from build123d import *

# Parameters (mm, degrees)
SKETCH1_R           = 7.9375
BOSS_EXTRUDE1_DEPTH = 19.05
SKETCH2_W           = 3.175
SKETCH2_H           = 3.446915699
BOSS_EXTRUDE2_DEPTH = 19.05
SKETCH3_R           = 5.5626
CUT_EXTRUDE1_DEPTH  = 19.05


with BuildPart() as part:
    # Sketch1 → Boss-Extrude1 (new body)
    with BuildSketch(Plane(origin=(0, 0, 0), x_dir=(0, 0, -1), z_dir=(1, 0, 0))):
        Circle(SKETCH1_R)
    extrude(amount=BOSS_EXTRUDE1_DEPTH)

    # Sketch2 → Boss-Extrude2 (add)
    with BuildSketch(Plane.ZY):
        with Locations((0, 7.636442151)):
            Rectangle(SKETCH2_W, SKETCH2_H)
        with Locations((0, -7.636442151)):
            Rectangle(SKETCH2_W, SKETCH2_H)
    extrude(amount=-BOSS_EXTRUDE2_DEPTH)

    # Sketch3 → Cut-Extrude1 (cut)
    with BuildSketch(Plane.ZY):
        Circle(SKETCH3_R)
    extrude(amount=-CUT_EXTRUDE1_DEPTH, mode=Mode.SUBTRACT)


solid = part.part
For this review, take the finished solid that the model builds, in its own axes (mm). A direction names the side the tool comes from. Round coordinates to 2 decimals unless told otherwise and drop trailing zeros. Order: outer loops, then holes, each group sorted by start corner. A loop starts at its lowest first (then second) coordinate and runs counter-clockwise, first axis right, second up. Notation, with made-up numbers: M 19.25,52 L 61.25,52 A13 ccw 61.25,63 Z; hole C 14.5,-15.75 d8. An arc over 180 degrees is marked long. Write each question's results on one line, items separated by ' | '. Start each with the question number.
1. Add section B-B (y = 0). State the section outline as (x, z) points, then the cut area to 3 significant figures.
2. Add section A-A (z = 0). State the section outline as (x, y) points.
3. To check wall thickness, follow L1, parallel to Y at x = 13, z = 0; L2, parallel to Z at x = 6.5, y = -0.25; L3, parallel to Z at x = 6.75, y = -8.5. State the ranges of each line that lie inside material, in increasing order. Write a range as [from, to].
4. Add section D-D (y = -6.75). State the section outline as (x, z) points, then the cut area to 3 significant figures.
5. Draft analysis for pull direction Z (two halves, no side actions). For faces 4 (the face through (9, 9, -1.588)), 5 (the face through (9, -9, 1.588)), 6 (the face through (9.392, 1.671, 5.306)), state which applies: pulls with the +Z half, pulls with the -Z half, needs draft (parallel to the pull), parting line crosses it, or undercut.
6. Tool access review of faces 1 (the face through (9, -9, -1.588)), 2 (the face through (9, 9, 1.588)), 3 (the face through (9.392, 0.152, 7.936)): name each direction out of +Z, -Z, +X, -X, +Y, -Y from which nothing blocks a thin tool from reaching the whole face with its end or side.
7. Clearance check with flat-ended pins moving along their axes: pin 1 Ø1 at (x, z) = (16.5, 6) entering from +Y; pin 2 Ø3 at (x, y) = (10.5, 2) entering from -Z; pin 3 Ø5 at (x, y) = (9, -7) entering from -Z. State where each tip first meets the part, or that it passes through.
Output values:
1) outline: M 0,-7.94 L 19.05,-7.94 L 19.05,-5.56 L 0,-5.56 Z; M 0,5.56 L 19.05,5.56 L 19.05,7.94 L 0,7.94 Z | area: 90.5 mm^2
2) outline: M 0,-9.36 L 19.05,-9.36 L 19.05,-5.56 L 0,-5.56 Z; M 0,5.56 L 19.05,5.56 L 19.05,9.36 L 0,9.36 Z
3) L1: [-9.36, -5.56], [5.56, 9.36] | L2: [-7.93, -5.56], [5.56, 7.93] | L3: [-1.59, 1.59]
4) outline: M 0,-4.18 L 19.05,-4.18 L 19.05,4.18 L 0,4.18 Z | area: 159 mm^2
5) face 4: pulls with the -Z half | face 5: pulls with the +Z half | face 6: undercut
6) face 1: -Z, +X, -X, -Y | face 2: +Z, +X, -X, +Y | face 3: +Z, +X, -X
7) pin 1: y = 5.72 | pin 2: z = -7.92 | pin 3: z = -6.54
